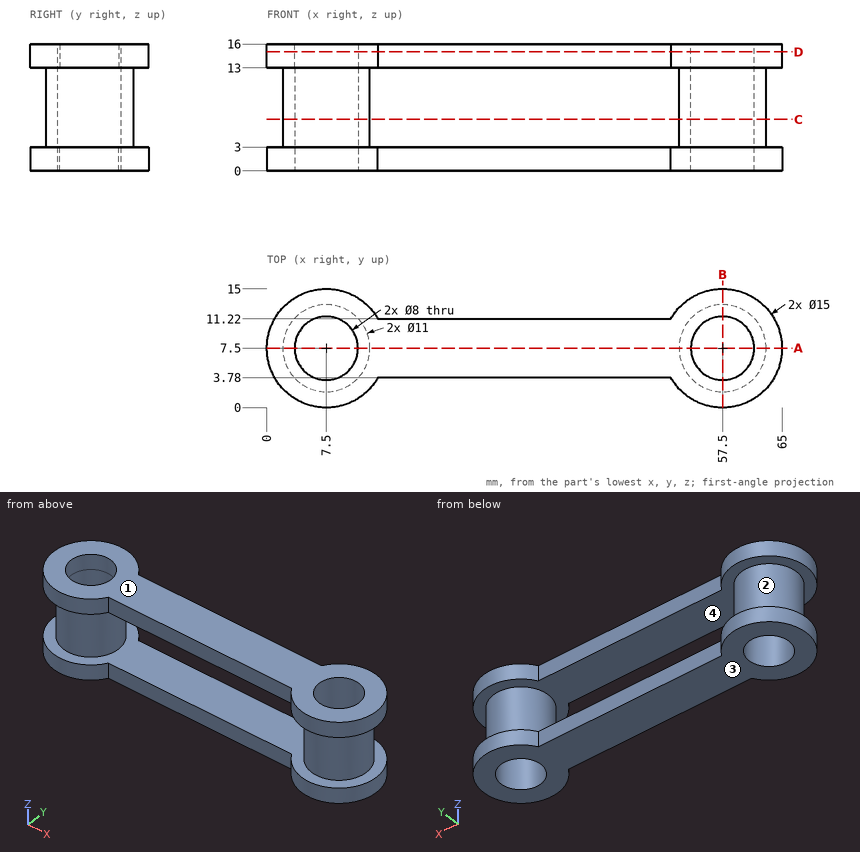
Input: dimensioned drawing with shaded views. Units: mm. Origin: part minimum x, y, z. A direction names the side the tool comes from. Coordinates: 2 decimals unless noted, no trailing zeros. Order: outer loops, then holes, each group sorted by start corner. A loop starts at its lowest first (then second) coordinate and runs counter-clockwise, first axis right, second up. Notation, with made-up numbers: (-20.5, 46.25) -> (2.5, 46.25) arc R16 ccw to (2.5, 64.25) -> close; hole circle Ø4 at (-31, -29.5). An arc over 180 degrees is marked (long way). Use CSV: the item, a comma, the result in double quotes.
1) Section A-A on y = 7.5. Output: boundary loops of the cut face in (x, z).
Findings:
outline,"(0, 0) -> (3.5, 0) -> (3.5, 16) -> (0, 16) -> (0, 13) -> (2, 13) -> (2, 3) -> (0, 3) -> close; (11.5, 0) -> (53.5, 0) -> (53.5, 16) -> (11.5, 16) -> close; (61.5, 0) -> (65, 0) -> (65, 3) -> (63, 3) -> (63, 13) -> (65, 13) -> (65, 16) -> (61.5, 16) -> close; hole (13, 3) -> (52, 3) -> (52, 13) -> (13, 13) -> close"
2) Line query: line 1 (X direction, y = 7.5, z = 5); line 2 (Y direction, x = 7.5, z = 14.45); line 3 (Z direction, x = 23, y = 8.75). Output: solid intervals per line, ascending.
Findings:
line 1,"x = 2 to 3.5, 11.5 to 13, 52 to 53.5, 61.5 to 63"
line 2,"y = 0 to 3.5, 11.5 to 15"
line 3,"z = 0 to 3, 13 to 16"
3) Mould query, pull axis X, two halves, no side actions, for the marked faces 1 and 2. Classes: +X half, -X half, draft (parallel to the pull), parting line (faces both ways), or undercut.
Findings:
face 1,"draft"
face 2,"undercut"
4) Section C-C on z = 6.5. Output: boundary loops of the cut face in (x, y).
Findings:
outline,"circle Ø11 at (7.5, 7.5); circle Ø11 at (57.5, 7.5); hole circle Ø8 at (7.5, 7.5); hole circle Ø8 at (57.5, 7.5)"
5) Section B-B on x = 57.5. Output: boundary loops of the cut face in (y, z).
Findings:
outline,"(0, 0) -> (3.5, 0) -> (3.5, 16) -> (0, 16) -> (0, 13) -> (2, 13) -> (2, 3) -> (0, 3) -> close; (11.5, 0) -> (15, 0) -> (15, 3) -> (13, 3) -> (13, 13) -> (15, 13) -> (15, 16) -> (11.5, 16) -> close"
6) Access query for the marked faces 3 and 4. Directions: +Z, -Z, +X, -X, +Y, -Y. A direction counts if a zero-diameter tool reaches every point of the face in a straight line with its end or side. Return the directions, or none.
Findings:
face 3,"-Z, +X, -X, +Y, -Y"
face 4,"none"
7) Pin query (flat end, axial travel): pin 1 Ø2.5 at (x, z) = (33, 14) entering from +Y; pin 2 Ø7 at (x, y) = (7.5, 7.5) entering from +Z; pin 3 Ø1.5 at (x, z) = (27, 1) entering from -Y; pin 4 Ø6 at (y, z) = (5.5, 10.5) entering from -X. Return the tip coordinate at first contact, or that it passes through.
Findings:
pin 1,"stops at y = 11.22"
pin 2,"passes through"
pin 3,"stops at y = 3.78"
pin 4,"stops at x = 0.01"
8) Section D-D on z = 15. Output: boundary loops of the cut face in (x, y).
Findings:
outline,"(14.01, 3.78) -> (50.99, 3.78) arc R7.5 ccw (long way) to (50.99, 11.22) -> (14.01, 11.22) arc R7.5 ccw (long way) to start; hole circle Ø8 at (7.5, 7.5); hole circle Ø8 at (57.5, 7.5)"
